```python
from build123d import *

# Parameters (mm, degrees)
SKETCH_1_W          = 50
SKETCH_1_H          = 75
EXTRUDE_1_DEPTH     = 6
CUT_EXTRUDE_1_DEPTH = 46.467021015
M3X0_51_AT_2_COUNT  = 2
M3X0_51_AT_2_PITCH  = 31.5
M3X0_51_AT_3_COUNT  = 2
M3X0_51_AT_3_PITCH  = 63
SKETCH_6_W          = 10
SKETCH_6_H          = 75
CUT_EXTRUDE_2_DEPTH = 2
SKETCH_7_W          = 15
SKETCH_7_H          = 15
CUT_EXTRUDE_3_DEPTH = 46.467021015
FILLET_1_R          = 3


with BuildPart() as part:
    # Эскиз1 → Бобышка-Вытянуть1 (new body)
    with BuildSketch(Plane.XY):
        Rectangle(SKETCH_1_W, SKETCH_1_H)
    extrude(amount=EXTRUDE_1_DEPTH)

    # Эскиз2 → Вырез-Вытянуть1 (cut, through all)
    with BuildSketch(Plane.XY.offset(6)):
        with BuildLine():
            Line((16.75, 30.5), (16.75, -30.5))
            ThreePointArc((16.75, -30.5), (14, -33.25), (11.25, -30.5))
            Line((11.25, -30.5), (11.25, 30.5))
            ThreePointArc((11.25, 30.5), (14, 33.25), (16.75, 30.5))
        make_face()
    extrude(amount=-CUT_EXTRUDE_1_DEPTH, mode=Mode.SUBTRACT)

    # Эскиз4 → Отверстие обработанное метчиком M3x0.51 (revolve, cut)
    with BuildSketch(Plane(origin=(-25, 31.5, 3), x_dir=(0, 0, 1), z_dir=(0, 1, 0))):
        Polygon((0, 0), (0, 6.751075774), (1.25, 6), (1.25, 0), align=None)
    m3x0_51 = revolve(axis=Axis((-31.35, 31.5, 3), (1, 0, 0)), mode=Mode.SUBTRACT)

    # Отверстие обработанное метчиком M3x0.51 at 2: Отверстие обработанное метчиком M3x0.51 ×2
    with Locations(*[(0, -i * M3X0_51_AT_2_PITCH, 0) for i in range(1, M3X0_51_AT_2_COUNT)]):
        add(m3x0_51, mode=Mode.SUBTRACT)

    # Отверстие обработанное метчиком M3x0.51 at 3: Отверстие обработанное метчиком M3x0.51 ×2
    with Locations(*[(0, -i * M3X0_51_AT_3_PITCH, 0) for i in range(1, M3X0_51_AT_3_COUNT)]):
        add(m3x0_51, mode=Mode.SUBTRACT)

    # Зеркальное отражение1: Отверстие обработанное метчиком M3x0.51 across plane
    add(m3x0_51.mirror(Plane.ZY), mode=Mode.SUBTRACT)

    # Зеркальное отражение1 copy 1 sketch → Зеркальное отражение1 copy 1 (revolve, cut)
    with BuildSketch(Plane(origin=(25, 0, 3), x_dir=(0, 0, 1), z_dir=(0, 1, 0))):
        Polygon((0, 0), (0, -6.751075774), (1.25, -6), (1.25, 0), align=None)
    revolve(axis=Axis((31.35, 0, 3), (1, 0, 0)), mode=Mode.SUBTRACT)

    # Зеркальное отражение1 copy 2 sketch → Зеркальное отражение1 copy 2 (revolve, cut)
    with BuildSketch(Plane(origin=(25, -31.5, 3), x_dir=(0, 0, 1), z_dir=(0, 1, 0))):
        Polygon((0, 0), (0, -6.751075774), (1.25, -6), (1.25, 0), align=None)
    revolve(axis=Axis((31.35, -31.5, 3), (1, 0, 0)), mode=Mode.SUBTRACT)

    # Эскиз6 → Вырез-Вытянуть2 (cut)
    with BuildSketch(Plane.XY.offset(6)):
        with Locations((14, 0)):
            Rectangle(SKETCH_6_W, SKETCH_6_H)
    extrude(amount=-CUT_EXTRUDE_2_DEPTH, mode=Mode.SUBTRACT)

    # Эскиз7 → Вырез-Вытянуть3 (cut, through all)
    with BuildSketch(Plane.XY.offset(6)):
        with Locations((-11.5, -30)):
            Rectangle(SKETCH_7_W, SKETCH_7_H)
    extrude(amount=-CUT_EXTRUDE_3_DEPTH, mode=Mode.SUBTRACT)

    # Скругление1
    fillet_1_edges = [part.edges().sort_by_distance(p)[0] for p in [
        (-19, -37.5, 3),
        (-4, -22.5, 3),
        (-4, -37.5, 3),
        (-19, -22.5, 3),
    ]]
    fillet(fillet_1_edges, radius=FILLET_1_R)


solid = part.part
```
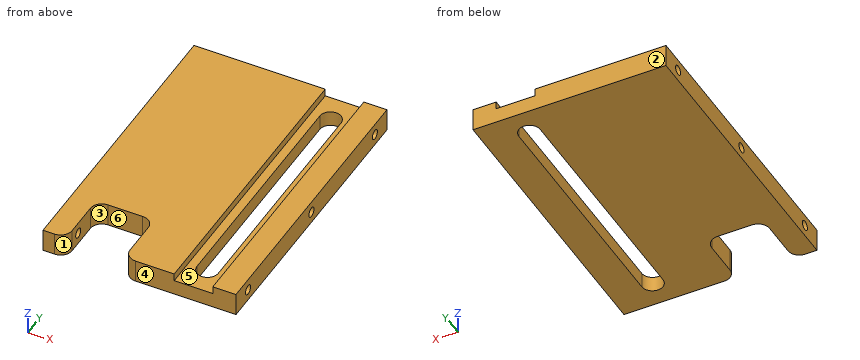
The model under review builds one solid part; all positions refer to its coordinate system, in mm. Face numbers are marked on the shaded views. A direction names the side the tool comes from. Coordinates: 2 decimals unless noted, no trailing zeros. Order: outer loops, then holes, each group sorted by start corner. A loop starts at its lowest first (then second) coordinate and runs counter-clockwise, first axis right, second up. Notation, with made-up numbers: M 32,75 L 56,75 A18 ccw 56,81 Z; hole C -22.75,65 d11. An arc over 180 degrees is marked long. One line per question, with ' | ' between items.
(1) Machinability: for the marked faces 4, 5 and 6, which of the approach directions +Z, -Z, +X, -X, +Y, -Y give a long, thin tool a straight path to every point of the face, cutting with its end or side? Answer none if there is none.
Geometry results:
face 4: +Z, -Z, +X, -X, -Y | face 5: +Z, +Y, -Y | face 6: +Z, -Z, -Y
(2) The part is to be moulded in two halves that separate along X. For the marked faces 1, 2 and 3, say which applies: +X half, -X half, draft (parallel to the pull), parting line (faces both ways), or undercut.
Geometry results:
face 1: undercut | face 2: draft | face 3: undercut
(3) Add section A-A, the plane x = 14. Write out the cut boundary in (y, z), then the cut area to 3 significant figures.
Geometry results:
outline: M -37.5,0 L -33.25,0 L -33.25,4 L -37.5,4 Z; M 33.25,0 L 37.5,0 L 37.5,4 L 33.25,4 Z | area: 34.0 mm²
(4) Add section C-C, the plane x = -12. Write out the cut boundary in (y, z), then the cut area to 3 significant figures.
Geometry results:
outline: M -22.5,0 L 37.5,0 L 37.5,6 L -22.5,6 Z | area: 360 mm²
(5) For probe 1 along Y at (x, z) = (23.7, 3); probe 2 along X at (y, z) = (-29, 3.4); probe 3 along Z at (x, y) = (-22, 0), list the stretches that pass through material, from the lowest coordinate up. Write a range as from..to.
Geometry results:
probe 1: y = -37.5..-32.75, -30.25..-1.25, 1.25..30.25, 32.75..37.5 | probe 2: x = -25..-19, -4..11.25, 16.75..25 | probe 3: z = 0..1.75, 4.25..6
(6) Add section B-B, the plane y = -8.5. Write out the cut boundary in (x, z), then the cut area to 3 significant figures.
Geometry results:
outline: M -25,0 L 11.25,0 L 11.25,4 L 9,4 L 9,6 L -25,6 Z; M 16.75,0 L 25,0 L 25,6 L 19,6 L 19,4 L 16.75,4 Z | area: 258 mm²
(7) Insertion check: pin 1 (2 mm diameter, centred on y = 31.5, z = 3, fed in from -X); pin 2 (5 mm diameter, centred on x = 15.5, y = 7.5, fed in from +Z); pin 3 (2 mm diameter, centred on y = -31.5, z = 3, fed in from +X). Each pin has a flat end and moves straight along its axis. Give the tip position at first contact, or say it passes through.
Geometry results:
pin 1: stops at x = -18.85 | pin 2: stops at z = 4 | pin 3: stops at x = 18.85
